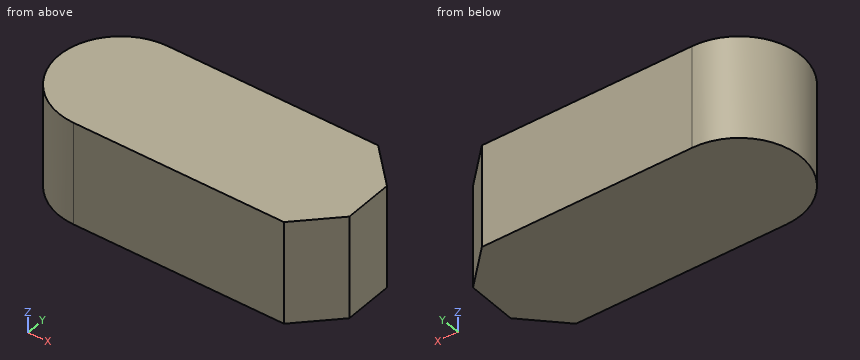
```python
from build123d import *

# Parameters (mm, degrees)
F1_DEPTH = 25


with BuildPart() as f1:
    # F0 (on Top) → F1 (new body)
    with BuildSketch(Plane.XY):
        with BuildLine():
            ThreePointArc((0, 30), (-15, 15), (0, 0))
            Line((0, 0), (51, 0))
            Line((51, 0), (60, 9))
            Line((60, 9), (60, 21))
            Line((60, 21), (51, 30))
            Line((51, 30), (0, 30))
        make_face()
    extrude(amount=F1_DEPTH)


solid = f1.part
```
Design review of the part built by this model. Coordinates are the model's own, in mm. Give positions to 0.01 mm unless a question says otherwise; leave off trailing zeros. Loops run counter-clockwise (first coordinate to the right, second up) from the corner with the lowest first, then second, coordinate; pieces in that order, holes last. Notation, with made-up numbers: M 73,19 L 102,19 A15 cw 102,43 Z; hole C -35.75,59 d10. An arc over 180 degrees is marked long. Return JSON: item names as keys, results as strings. Group by question number.
Item 1: Insertion check: pin 1 Ø2 at (y, z) = (9.5, 5) entering from -X; pin 2 Ø1.5 at (y, z) = (22, 19.5) entering from +X; pin 3 Ø3 at (y, z) = (5.5, 3.5) entering from +X. Each pin has a flat end and moves straight along its axis. Give the tip position at first contact, or say it passes through.
Item 2: For probe 1 along X at (y, z) = (18.5, 11.75); probe 2 along X at (y, z) = (13.75, 12.25); probe 3 along Y at (x, z) = (-11.5, 19.25), list the stretches that pass through material, from the lowest coordinate up.
Item 3: We need section A-A (z = 7). Give the boundary of the cut face in (x, y).
Item 4: We need section B-B (y = 24.25). Give the boundary of the cut face in (x, z), and give its area (3 significant figures).
Output:
{
 "1": {"pin 1": "stops at x = -14.31", "pin 2": "stops at x = 59.75", "pin 3": "stops at x = 58"},
 "2": {"probe 1": "x = -14.59 to 60", "probe 2": "x = -14.95 to 60", "probe 3": "y = 5.37 to 24.63"},
 "3": {"outline": "M 0,0 L 51,0 L 60,9 L 60,21 L 51,30 L 0,30 A15 ccw Z"},
 "4": {"outline": "M -11.81,0 L 56.75,0 L 56.75,25 L -11.81,25 Z", "area": "1,710 mm^2"}
}
